Could you check a few things on this model? Use its own coordinates, in mm. A direction names the side the tool comes from. Round coordinates to 2 decimals unless told otherwise and drop trailing zeros. Write each loop counter-clockwise with the first axis right and the second up, starting at its lowest first coordinate (ties: lowest second). Pieces come first, ordered by that corner, then holes. Notation, with made-up numbers: (65.5, -29.5) - (86.5, -29.5) arc R19 cw to (86.5, -9.5) - close; hole circle Ø2 at (-8, -16). An arc over 180 degrees is marked (long way). Write each question's results on one line, items separated by ' | '. Start each with the question number.
(1) Imagine slicing it at B-B on x = 1.5. Write out the boundary of the cut face in (y, z).
(2) Please list where these lines run through material, in increasing order: line 1 (Y direction, x = 1.5, z = 0); line 2 (Y direction, x = 3.85, z = 0); line 3 (X direction, y = -1.5, z = 8.75). Write a range as [from, to].
(3) Imagine slicing it at A-A on x = 4.75. Write out the boundary of the cut face in (y, z).
(4) On a 3-axis mill with a long thin cutter (end or side, diameter ignored), from which of +Z, -Z, +X, -X, +Y, -Y can I reach the whole of each face in a straight line? I mean faces 4 (the flat face through (5.3, 0, 0)), 5 (the flat face through (3.3, 6, -5)), 6 (the cylindrical face through (1.63, 0.53, 11.99)). Say none if no direction works.
(5) For P1, Ø4, axis at x = 9, y = -2.5, coming from the -Z side; P2, Ø3, axis at x = 11.5, z = -6, coming from the -Y side; P3, Ø4, axis at x = 5.5, y = 6.5, coming from the -Z side, each with a flat end and sliding along its axis, tell me the tip position at first contact or that it passes through.
(6) Imagine slicing it at C-C on z = 10.75. Write out the boundary of the cut face in (x, y), then the cut area to 3 significant figures.
(7) Thinking about a two-plate mould opening in X: for faces 1 (the cylindrical face through (4.286, 0.33, 7.493)), 2 (the cylindrical face through (6.29, -9.76, 2.17)), 3 (the flat face through (13.3, 0, 0)), which applies, +X half, -X half, draft (parallel to the pull), parting line (faces both ways), or undercut?
```python
from build123d import *

# Parameters (mm, degrees)
SKETCH_2_R      = 12
SKETCH_2_R_2    = 4
EXTRUDE_1_DEPTH = 3.3
SKETCH_3_R      = 7.5
SKETCH_3_R_2    = 4
EXTRUDE_2_DEPTH = 2
SKETCH_4_R      = 10
EXTRUDE_3_DEPTH = 8
FILLET_1_R      = 6


with BuildPart() as part:
    # Эскиз2 → Бобышка-Вытянуть1 (new body)
    with BuildSketch(Plane(origin=(0, 0, 0), x_dir=(0, 0, -1), z_dir=(1, 0, 0))):
        Circle(SKETCH_2_R)
        Circle(SKETCH_2_R_2, mode=Mode.SUBTRACT)
    extrude(amount=EXTRUDE_1_DEPTH)

    # Эскиз3 → Бобышка-Вытянуть2 (add)
    with BuildSketch(Plane(origin=(3.3, 0, 0), x_dir=(0, 0, -1), z_dir=(1, 0, 0))):
        Circle(SKETCH_3_R)
        Circle(SKETCH_3_R_2, mode=Mode.SUBTRACT)
    extrude(amount=EXTRUDE_2_DEPTH)

    # Эскиз4 → Бобышка-Вытянуть3 (add)
    with BuildSketch(Plane(origin=(5.3, 0, 0), x_dir=(0, 0, -1), z_dir=(1, 0, 0))):
        Circle(SKETCH_4_R)
    extrude(amount=EXTRUDE_3_DEPTH)

    # Скругление1
    fillet_1_edges = [part.edges().sort_by_distance(p)[0] for p in [
        (13.3, 0, 10),
    ]]
    fillet(fillet_1_edges, radius=FILLET_1_R)


solid = part.part
```
Response:
1) outline: circle Ø24 at (0, 0); hole circle Ø8 at (0, 0)
2) line 1: [-12, -4], [4, 12] | line 2: [-7.5, -4], [4, 7.5] | line 3: [0, 3.3], [5.3, 10.79]
3) outline: circle Ø15 at (0, 0); hole circle Ø8 at (0, 0)
4) face 4: -X | face 5: none | face 6: +X, -X
5) P1: z = -9.94 | P2: y = -7.66 | P3: z = -8.93
6) outline: (0, -5.33) - (3.3, -5.33) - (3.3, 5.33) - (0, 5.33) - close | area: 35.2 mm²
7) face 1: undercut | face 2: draft | face 3: +X half
